Check sheet for the modelled part. Datum: model origin and axes. Units: mm. Face numbers are marked on the shaded views. A direction names the side the tool comes from. Round coordinates to 2 decimals unless told otherwise and drop trailing zeros. Write each loop counter-clockwise with the first axis right and the second up, starting at its lowest first coordinate (ties: lowest second). Pieces come first, ordered by that corner, then holes. Notation, with made-up numbers: (41.5, 10.5) - (46.5, 10.5) arc R20 ccw to (46.5, 20.5) - close; hole circle Ø2 at (-40, 63.5). An arc over 180 degrees is marked (long way). Answer as a JSON object with one key per item and string values. Group by question number.
Item 1: Set-up check for the marked faces 1, 2 and 3: record each of +Z, -Z, +X, -X, +Y, -Y from which the full face is reachable in a straight line by a thin tool's end or side.
Item 2: Release check for a two-part mould opening along Z. For the marked faces 4, 5 and 6 record: pulls with the +Z half, pulls with the -Z half, needs draft (parallel to the pull), parting line crosses it, or undercut.
Item 3: Sectioned sample at C-C on z = 0. Record the boundary of the cut face in (x, y) (3 decimals), plus the area to 3 significant figures.
Item 4: Sectioned sample at B-B on y = -12. Record the boundary of the cut face in (x, z).
Item 5: Sectioned sample at D-D on y = 26. Record the boundary of the cut face in (x, z), plus the area to 3 significant figures.
Item 6: Thickness scan on line 1 (X direction, y = 33.25, z = 0); line 2 (X direction, y = 10, z = 5); line 3 (X direction, y = -14, z = -11). Record the ranges inside material, lowest first.
Item 7: Sectioned sample at A-A on x = 0. Record the boundary of the cut face in (y, z), plus the area to 3 significant figures.
Item 8: Gauge pin test, flat ends, axial feed: P1, Ø10, axis at y = -9.5, z = -21, coming from the +X side; P2, Ø21.5, axis at x = 0, y = 0, coming from the -Z side; P3, Ø6, axis at y = 13.5, z = 16, coming from the +X side. Record the tip position at first contact, or that the pin passes through.
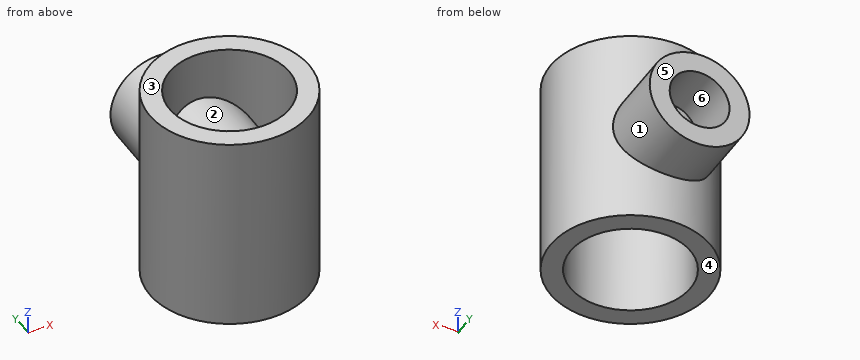
```python
from build123d import *

# Parameters (mm, degrees)
CROQUIS1_R              = 24
CROQUIS1_R_2            = 18
SALIENTE_EXTRUIR1_DEPTH = 30
CROQUIS2_R              = 15
CROQUIS2_R_2            = 9
SALIENTE_EXTRUIR2_DEPTH = 40


with BuildPart() as part:
    # Croquis1 → Saliente-Extruir1 (new, symmetric)
    with BuildSketch(Plane.XY):
        Circle(CROQUIS1_R)
        Circle(CROQUIS1_R_2, mode=Mode.SUBTRACT)
    extrude(amount=SALIENTE_EXTRUIR1_DEPTH, both=True)

    # Croquis2 → Saliente-Extruir2 (add)
    with BuildSketch(Plane(origin=(0, 0, 0), x_dir=(1, 0, 0), z_dir=(0, 1, 0))):
        with Locations(Location((0, 0, 0), (0, 0, 90))):
            Circle(CROQUIS2_R)
        with Locations(Location((0, 0, 0), (0, 0, 90))):
            Circle(CROQUIS2_R_2, mode=Mode.SUBTRACT)
    extrude(amount=SALIENTE_EXTRUIR2_DEPTH)


solid = part.part
```
Completed:
{
 "1": {"face 1": "+Y", "face 2": "none", "face 3": "+Z, +X, -X, +Y, -Y"},
 "2": {"face 4": "pulls with the -Z half", "face 5": "needs draft", "face 6": "undercut"},
 "3": {"outline": "(-15, 18.735) arc R24 ccw (long way) to (15, 18.735) - (15, 40) - (9, 40) - (9, 22.249) arc R24 ccw to (-9, 22.249) - (-9, 40) - (-15, 40) - close; hole (-15, 0) - (-15, 9.95) arc R18 ccw (long way) to (15, 9.95) - (15, 0) - (9, 0) - (9, 15.588) arc R18 ccw to (-9, 15.588) - (-9, 0) - close", "area": "1,180 mm²"},
 "4": {"outline": "(-20.78, -30) - (-13.42, -30) - (-13.42, 30) - (-20.78, 30) - close; (13.42, -30) - (20.78, -30) - (20.78, 30) - (13.42, 30) - close"},
 "5": {"outline": "circle Ø30 at (0, 0); hole circle Ø18 at (0, 0)", "area": "452 mm²"},
 "6": {"line 1": "-15 to -9, 9 to 15", "line 2": "-21.82 to -14.97, -14.14 to -7.48, 7.48 to 14.14, 14.97 to 21.82", "line 3": "-19.49 to -11.31, 11.31 to 19.49"},
 "7": {"outline": "(-24, -30) - (-18, -30) - (-18, 30) - (-24, 30) - close; (0, -15) - (18, -15) - (18, -30) - (24, -30) - (24, -15) - (40, -15) - (40, -9) - (24, -9) - (24, 9) - (40, 9) - (40, 15) - (24, 15) - (24, 30) - (18, 30) - (18, 15) - (0, 15) - (0, 9) - (18, 9) - (18, -9) - (0, -9) - close", "area": "1,130 mm²"},
 "8": {"P1": "x = 23.57", "P2": "z = -15", "P3": "x = 21.58"}
}
